Check sheet for the modelled part. Datum: model origin and axes. Units: mm. A direction names the side the tool comes from. Round coordinates to 2 decimals unless told otherwise and drop trailing zeros. Write each loop counter-clockwise with the first axis right and the second up, starting at its lowest first coordinate (ties: lowest second). Pieces come first, ordered by that corner, then holes.
Item 1: Tool access check on faces 4 (the flat face through (5, 75, -301.763)), 5 (the flat face through (-5, 149.263, -317)), 6 (the flat face through (395, 148.527, -4)), 7 (the flat face through (-6, 75, 301.763)), 8 (the flat face through (379.263, 75, 4)). Record the directions out of +Z, -Z, +X, -X, +Y, -Y that give a thin tool (end or side, any length) a straight path to the whole face; none if there is none.
Item 2: Material ranges on line 1 (Z direction, x = 344, y = 81); line 2 (X direction, y = 100.5, z = -54); line 3 (Y direction, x = 33.5, z = 247), recorded low to high.
Item 3: Cross-section at D-D on x = 291.5. Enter the section's corners in (y, z), plus the area to 3 significant figures.
Item 4: Cross-section at B-B on y = 35. Enter the section's corners in (x, z), plus the area to 3 significant figures.
Item 5: Cross-section at A-A on x = 0. Enter the section's corners in (y, z).
Item 6: Release check for a two-part mould opening along X. For faces 1 (the cylindrical face through (24.03, -0.363, -66.194)), 2 (the flat face through (-5, 148.527, -318)), 3 (the flat face through (380, 73, 4)) record: +X half, -X half, draft (parallel to the pull), parting line (faces both ways), or undercut.
Item 7: Cross-section at C-C on z = -142.5. Enter the section's corners in (x, y), plus the area to 3 significant figures.
Item 8: Go/stop test with flat-tipped pins: pin 1 Ø10 at (y, z) = (114, 121.5) entering from +X; pin 2 Ø1 at (x, y) = (-195, 82) entering from +Z; pin 3 Ø1 at (x, y) = (312.5, 131) entering from -Z. Record where each tip stops, or that it passes through.
from build123d import *

# Parameters (mm, degrees)
SKETCH1_W                    = 760
SKETCH1_H                    = 605
SKETCH1_R                    = 80
BASE_FLANGE1_DEPTH           = 0.7366
EDGE_FLANGE1_STRIP_W         = 4.4196
EDGE_FLANGE1_STRIP_H         = 0.7366
EDGE_FLANGE1_STRIP_CUT_DEPTH = 605
EDGE_FLANGE1_DEPTH           = 605
EDGE_FLANGE2_STRIP_W         = 4.4196
EDGE_FLANGE2_STRIP_H         = 0.7366
EDGE_FLANGE2_STRIP_CUT_DEPTH = 758.5268
EDGE_FLANGE2_DEPTH           = 758.5268
EDGE_FLANGE3_STRIP_W         = 4.4196
EDGE_FLANGE3_STRIP_H         = 0.7366
EDGE_FLANGE3_STRIP_CUT_DEPTH = 603.5268
EDGE_FLANGE3_DEPTH           = 603.5268
EDGE_FLANGE4_STRIP_W         = 4.4196
EDGE_FLANGE4_STRIP_H         = 0.7366
EDGE_FLANGE4_STRIP_CUT_DEPTH = 757.0536
EDGE_FLANGE4_DEPTH           = 757.0536
EDGE_FLANGE5_STRIP_W         = 4.4196
EDGE_FLANGE5_STRIP_H         = 0.7366
EDGE_FLANGE5_STRIP_CUT_DEPTH = 758.5268
EDGE_FLANGE5_DEPTH           = 758.5268
EDGE_FLANGE6_STRIP_W         = 4.4196
EDGE_FLANGE6_STRIP_H         = 0.7366
EDGE_FLANGE6_STRIP_CUT_DEPTH = 603.5268
EDGE_FLANGE6_DEPTH           = 603.5268
EDGE_FLANGE7_STRIP_W         = 4.4196
EDGE_FLANGE7_STRIP_H         = 0.7366
EDGE_FLANGE7_STRIP_CUT_DEPTH = 757.0536
EDGE_FLANGE7_DEPTH           = 757.0536
EDGE_FLANGE8_STRIP_W         = 4.4196
EDGE_FLANGE8_STRIP_H         = 0.7366
EDGE_FLANGE8_STRIP_CUT_DEPTH = 605
EDGE_FLANGE8_DEPTH           = 605


# Sheet-metal steps are written as plain solids
with BuildPart() as part:
    # Sketch1 → Base-Flange1 (new body)
    with BuildSketch(Plane(origin=(0, 0, 0), x_dir=(1, 0, 0), z_dir=(0, 1, 0))):
        Rectangle(SKETCH1_W, SKETCH1_H)
        with Locations(Location((0, 142.5, 0), (0, 0, 270))):
            Circle(SKETCH1_R, mode=Mode.SUBTRACT)
    extrude(amount=-BASE_FLANGE1_DEPTH)

    # Edge-Flange1 strip (across the edge) → Edge-Flange1 strip cut (cut)
    with BuildSketch(Plane(origin=(380, 0, 302.5), x_dir=(-1, 0, 0), z_dir=(0, 0, -1))):
        with Locations((-0.7366, -0.3683)):
            Rectangle(EDGE_FLANGE1_STRIP_W, EDGE_FLANGE1_STRIP_H)
    extrude(amount=EDGE_FLANGE1_STRIP_CUT_DEPTH, mode=Mode.SUBTRACT)

    # Edge-Flange1 section (across the edge) → Edge-Flange1 (add)
    with BuildSketch(Plane(origin=(380, 0, 302.5), x_dir=(-1, 0, 0), z_dir=(0, 0, -1))):
        with BuildLine():
            Line((0, 0.7366), (0, 149.2634))
            Line((0, 149.2634), (0.7366, 149.2634))
            Line((0.7366, 149.2634), (0.7366, 0.7366))
            ThreePointArc((0.7366, 0.7366), (0.952345145, 0.215745145), (1.4732, 0))
            Line((1.4732, 0), (1.4732, -0.7366))
            ThreePointArc((1.4732, -0.7366), (0.43149029, -0.30510971), (0, 0.7366))
        make_face()
    extrude(amount=EDGE_FLANGE1_DEPTH)

    # Edge-Flange2 strip (across the edge) → Edge-Flange2 strip cut (cut)
    with BuildSketch(Plane(origin=(-380, 0, 302.5), x_dir=(0, 0, -1), z_dir=(1, 0, 0))):
        with Locations((-0.7366, -0.3683)):
            Rectangle(EDGE_FLANGE2_STRIP_W, EDGE_FLANGE2_STRIP_H)
    extrude(amount=EDGE_FLANGE2_STRIP_CUT_DEPTH, mode=Mode.SUBTRACT)

    # Edge-Flange2 section (across the edge) → Edge-Flange2 (add)
    with BuildSketch(Plane(origin=(-380, 0, 302.5), x_dir=(0, 0, -1), z_dir=(1, 0, 0))):
        with BuildLine():
            Line((0, 0.7366), (0, 149.2634))
            Line((0, 149.2634), (0.7366, 149.2634))
            Line((0.7366, 149.2634), (0.7366, 0.7366))
            ThreePointArc((0.7366, 0.7366), (0.952345145, 0.215745145), (1.4732, 0))
            Line((1.4732, 0), (1.4732, -0.7366))
            ThreePointArc((1.4732, -0.7366), (0.43149029, -0.30510971), (0, 0.7366))
        make_face()
    extrude(amount=EDGE_FLANGE2_DEPTH)

    # Edge-Flange3 strip (across the edge) → Edge-Flange3 strip cut (cut)
    with BuildSketch(Plane(origin=(-380, 0, -302.5), x_dir=(1, 0, 0), z_dir=(0, 0, 1))):
        with Locations((-0.7366, -0.3683)):
            Rectangle(EDGE_FLANGE3_STRIP_W, EDGE_FLANGE3_STRIP_H)
    extrude(amount=EDGE_FLANGE3_STRIP_CUT_DEPTH, mode=Mode.SUBTRACT)

    # Edge-Flange3 section (across the edge) → Edge-Flange3 (add)
    with BuildSketch(Plane(origin=(-380, 0, -302.5), x_dir=(1, 0, 0), z_dir=(0, 0, 1))):
        with BuildLine():
            Line((0, 0.7366), (0, 149.2634))
            Line((0, 149.2634), (0.7366, 149.2634))
            Line((0.7366, 149.2634), (0.7366, 0.7366))
            ThreePointArc((0.7366, 0.7366), (0.952345145, 0.215745145), (1.4732, 0))
            Line((1.4732, 0), (1.4732, -0.7366))
            ThreePointArc((1.4732, -0.7366), (0.43149029, -0.30510971), (0, 0.7366))
        make_face()
    extrude(amount=EDGE_FLANGE3_DEPTH)

    # Edge-Flange4 strip (across the edge) → Edge-Flange4 strip cut (cut)
    with BuildSketch(Plane(origin=(378.5268, 0, -302.5), x_dir=(0, 0, 1), z_dir=(-1, 0, 0))):
        with Locations((-0.7366, -0.3683)):
            Rectangle(EDGE_FLANGE4_STRIP_W, EDGE_FLANGE4_STRIP_H)
    extrude(amount=EDGE_FLANGE4_STRIP_CUT_DEPTH, mode=Mode.SUBTRACT)

    # Edge-Flange4 section (across the edge) → Edge-Flange4 (add)
    with BuildSketch(Plane(origin=(378.5268, 0, -302.5), x_dir=(0, 0, 1), z_dir=(-1, 0, 0))):
        with BuildLine():
            Line((0, 0.7366), (0, 149.2634))
            Line((0, 149.2634), (0.7366, 149.2634))
            Line((0.7366, 149.2634), (0.7366, 0.7366))
            ThreePointArc((0.7366, 0.7366), (0.952345145, 0.215745145), (1.4732, 0))
            Line((1.4732, 0), (1.4732, -0.7366))
            ThreePointArc((1.4732, -0.7366), (0.43149029, -0.30510971), (0, 0.7366))
        make_face()
    extrude(amount=EDGE_FLANGE4_DEPTH)

    # Edge-Flange5 strip (across the edge) → Edge-Flange5 strip cut (cut)
    with BuildSketch(Plane(origin=(378.5268, 149.2634, 302.5), x_dir=(0, -1, 0), z_dir=(-1, 0, 0))):
        with Locations((-0.7366, -0.3683)):
            Rectangle(EDGE_FLANGE5_STRIP_W, EDGE_FLANGE5_STRIP_H)
    extrude(amount=EDGE_FLANGE5_STRIP_CUT_DEPTH, mode=Mode.SUBTRACT)

    # Edge-Flange5 section (across the edge) → Edge-Flange5 (add)
    with BuildSketch(Plane(origin=(378.5268, 149.2634, 302.5), x_dir=(0, -1, 0), z_dir=(-1, 0, 0))):
        with BuildLine():
            Line((0, 0.7366), (0, 29.2634))
            Line((0, 29.2634), (0.7366, 29.2634))
            Line((0.7366, 29.2634), (0.7366, 0.7366))
            ThreePointArc((0.7366, 0.7366), (0.952345145, 0.215745145), (1.4732, 0))
            Line((1.4732, 0), (1.4732, -0.7366))
            ThreePointArc((1.4732, -0.7366), (0.43149029, -0.30510971), (0, 0.7366))
        make_face()
    extrude(amount=EDGE_FLANGE5_DEPTH)

    # Edge-Flange6 strip (across the edge) → Edge-Flange6 strip cut (cut)
    with BuildSketch(Plane(origin=(-380, 149.2634, 301.0268), x_dir=(0, -1, 0), z_dir=(0, 0, -1))):
        with Locations((-0.7366, -0.3683)):
            Rectangle(EDGE_FLANGE6_STRIP_W, EDGE_FLANGE6_STRIP_H)
    extrude(amount=EDGE_FLANGE6_STRIP_CUT_DEPTH, mode=Mode.SUBTRACT)

    # Edge-Flange6 section (across the edge) → Edge-Flange6 (add)
    with BuildSketch(Plane(origin=(-380, 149.2634, 301.0268), x_dir=(0, -1, 0), z_dir=(0, 0, -1))):
        with BuildLine():
            Line((0, 0.7366), (0, 29.2634))
            Line((0, 29.2634), (0.7366, 29.2634))
            Line((0.7366, 29.2634), (0.7366, 0.7366))
            ThreePointArc((0.7366, 0.7366), (0.952345145, 0.215745145), (1.4732, 0))
            Line((1.4732, 0), (1.4732, -0.7366))
            ThreePointArc((1.4732, -0.7366), (0.43149029, -0.30510971), (0, 0.7366))
        make_face()
    extrude(amount=EDGE_FLANGE6_DEPTH)

    # Edge-Flange7 strip (across the edge) → Edge-Flange7 strip cut (cut)
    with BuildSketch(Plane(origin=(-378.5268, 149.2634, -302.5), x_dir=(0, -1, 0), z_dir=(1, 0, 0))):
        with Locations((-0.7366, -0.3683)):
            Rectangle(EDGE_FLANGE7_STRIP_W, EDGE_FLANGE7_STRIP_H)
    extrude(amount=EDGE_FLANGE7_STRIP_CUT_DEPTH, mode=Mode.SUBTRACT)

    # Edge-Flange7 section (across the edge) → Edge-Flange7 (add)
    with BuildSketch(Plane(origin=(-378.5268, 149.2634, -302.5), x_dir=(0, -1, 0), z_dir=(1, 0, 0))):
        with BuildLine():
            Line((0, 0.7366), (0, 29.2634))
            Line((0, 29.2634), (0.7366, 29.2634))
            Line((0.7366, 29.2634), (0.7366, 0.7366))
            ThreePointArc((0.7366, 0.7366), (0.952345145, 0.215745145), (1.4732, 0))
            Line((1.4732, 0), (1.4732, -0.7366))
            ThreePointArc((1.4732, -0.7366), (0.43149029, -0.30510971), (0, 0.7366))
        make_face()
    extrude(amount=EDGE_FLANGE7_DEPTH)

    # Edge-Flange8 strip (across the edge) → Edge-Flange8 strip cut (cut)
    with BuildSketch(Plane(origin=(380, 149.2634, -302.5), x_dir=(0, -1, 0), z_dir=(0, 0, 1))):
        with Locations((-0.7366, -0.3683)):
            Rectangle(EDGE_FLANGE8_STRIP_W, EDGE_FLANGE8_STRIP_H)
    extrude(amount=EDGE_FLANGE8_STRIP_CUT_DEPTH, mode=Mode.SUBTRACT)

    # Edge-Flange8 section (across the edge) → Edge-Flange8 (add)
    with BuildSketch(Plane(origin=(380, 149.2634, -302.5), x_dir=(0, -1, 0), z_dir=(0, 0, 1))):
        with BuildLine():
            Line((0, 0.7366), (0, 29.2634))
            Line((0, 29.2634), (0.7366, 29.2634))
            Line((0.7366, 29.2634), (0.7366, 0.7366))
            ThreePointArc((0.7366, 0.7366), (0.952345145, 0.215745145), (1.4732, 0))
            Line((1.4732, 0), (1.4732, -0.7366))
            ThreePointArc((1.4732, -0.7366), (0.43149029, -0.30510971), (0, 0.7366))
        make_face()
    extrude(amount=EDGE_FLANGE8_DEPTH)


solid = part.part
Response values:
1. face 4: +Y
1. face 5: +Z, -Z, +X, -X, +Y
1. face 6: +Z, -Z, +X, -Y
1. face 7: -X, +Y
1. face 8: +Z, -Z, +Y
2. line 1: z = -302.5 to -301.76, 301.76 to 302.5
2. line 2: x = -380 to -379.26, 379.26 to 380
2. line 3: y = -0.74 to 0
3. outline: (-0.74, -301.03) arc R1.47 ccw to (0.74, -302.5) - (147.79, -302.5) arc R0.74 cw to (148.53, -303.24) - (148.53, -331.76) - (149.26, -331.76) - (149.26, -303.24) arc R1.47 ccw to (147.79, -301.76) - (0.74, -301.76) arc R0.74 cw to (0, -301.03) - (0, 301.03) arc R0.74 cw to (0.74, 301.76) - (147.79, 301.76) arc R1.47 ccw to (149.26, 303.24) - (149.26, 331.76) - (148.53, 331.76) - (148.53, 303.24) arc R0.74 cw to (147.79, 302.5) - (0.74, 302.5) arc R1.47 ccw to (-0.74, 301.03) - close
3. area: 707 mm2
4. outline: (-380, -302.5) - (-379.26, -302.5) - (-379.26, 301.03) - (-380, 301.03) - close; (-380, 301.76) - (378.53, 301.76) - (378.53, 302.5) - (-380, 302.5) - close; (-378.53, -302.5) - (378.53, -302.5) - (378.53, -301.76) - (-378.53, -301.76) - close; (379.26, -302.5) - (380, -302.5) - (380, 302.5) - (379.26, 302.5) - close
4. area: 2,010 mm2
5. outline: (-0.74, -301.03) arc R1.47 ccw to (0.74, -302.5) - (147.79, -302.5) arc R0.74 cw to (148.53, -303.24) - (148.53, -331.76) - (149.26, -331.76) - (149.26, -303.24) arc R1.47 ccw to (147.79, -301.76) - (0.74, -301.76) arc R0.74 cw to (0, -301.03) - (0, -222.5) - (-0.74, -222.5) - close; (-0.74, -62.5) - (0, -62.5) - (0, 301.03) arc R0.74 cw to (0.74, 301.76) - (147.79, 301.76) arc R1.47 ccw to (149.26, 303.24) - (149.26, 331.76) - (148.53, 331.76) - (148.53, 303.24) arc R0.74 cw to (147.79, 302.5) - (0.74, 302.5) arc R1.47 ccw to (-0.74, 301.03) - close
6. face 1: undercut
6. face 2: draft
6. face 3: +X half
7. outline: (-409.26, 148.53) - (-380.74, 148.53) arc R0.74 cw to (-380, 147.79) - (-380, 0.74) arc R1.47 ccw to (-378.53, -0.74) - (-80, -0.74) - (-80, 0) - (-378.53, 0) arc R0.74 cw to (-379.26, 0.74) - (-379.26, 147.79) arc R1.47 ccw to (-380.74, 149.26) - (-409.26, 149.26) - close; (80, -0.74) - (378.53, -0.74) arc R1.47 ccw to (380, 0.74) - (380, 147.79) arc R0.74 cw to (380.74, 148.53) - (409.26, 148.53) - (409.26, 149.26) - (380.74, 149.26) arc R1.47 ccw to (379.26, 147.79) - (379.26, 0.74) arc R0.74 cw to (378.53, 0) - (80, 0) - close
7. area: 704 mm2
8. pin 1: stops at x = 380
8. pin 2: stops at z = 302.5
8. pin 3: stops at z = -302.5
